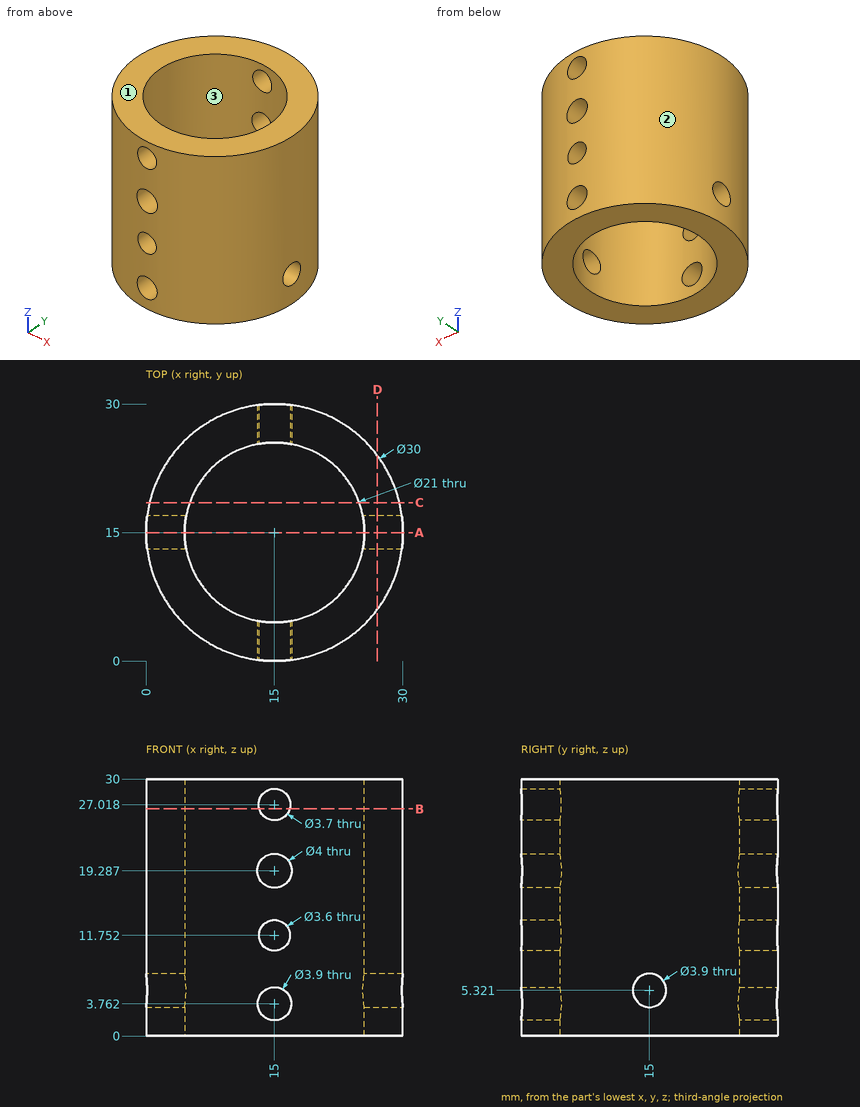
Study the drawing (mm; zero at the part's minimum x, y, z) and answer. Give positions to 0.01 mm unless a question says otherwise; leave off trailing zeros. Loops run counter-clockwise (first coordinate to the right, second up) from the corner with the lowest first, then second, coordinate; pieces in that order, holes last. Notation, with made-up numbers: (38.25, 78.25) -> (89.25, 78.25) arc R33 ccw to (89.25, 110.25) -> close; hole circle Ø7 at (-23.5, 35). An arc over 180 degrees is marked (long way). Write item = value, one per line. Start each with the question number.
(1) The mould has two halves that part along Y. Classify the marked faces 1, 2 and 3: +Y half, -Y half, draft (parallel to the pull), parting line (faces both ways), or undercut.
(2) Given pin 1 Ø12 at (y, z) = (7, 21) entering from -X; pin 2 Ø5 at (y, z) = (7, 17.5) entering from +X (1 decimal); pin 3 Ø1 at (x, z) = (9.5, 17.5) entering from -Y, each flat-ended and moving along its own axis, determine where each tip first touches the part or whether it passes through.
(3) Find the intervals of material crossed by probe 1 along X at (y, z) = (7, 21.5); probe 2 along X at (y, z) = (18.5, 22.5) (1 decimal); probe 3 along Y at (x, z) = (2.5, 4) (1 decimal), in increasing order. Write a range as from..to.
(4) Find section C-C on y = 18.5. Give the vertices of the cut face in (x, z).
(5) Find section B-B on z = 26.5. Give the vertices of the cut face in (x, y) (1 decimal).
(6) Find section A-A on y = 15. Give the vertices of the cut face in (x, z).
(7) Find section D-D on x = 27. Give the vertices of the cut face in (y, z), and give its area (3 significant figures).
From the geometry:
q1.face_1 = draft
q1.face_2 = parting line
q1.face_3 = undercut
q2.pin_1 = 0.13
q2.pin_2 = 29
q2.pin_3 = 0.86
q3.probe_1 = 2.31..8.2, 21.8..27.69
q3.probe_2 = 0.4..5.1, 24.9..29.6
q3.probe_3 = 6.7..13.6, 16.4..23.3
q4.outline = (0.41, 0) -> (5.1, 0) -> (5.1, 30) -> (0.41, 30) -> close; (24.9, 0) -> (29.59, 0) -> (29.59, 30) -> (24.9, 30) -> close
q5.outline = (13.2, 0.1) -> (13.2, 4.7) arc R10.5 cw to (13.2, 25.3) -> (13.2, 29.9) arc R15 ccw to start; (16.8, 0.1) arc R15 ccw to (16.8, 29.9) -> (16.8, 25.3) arc R10.5 cw to (16.8, 4.7) -> close
q6.outline = (0, 0) -> (4.5, 0) -> (4.5, 3.37) -> (0, 3.37) -> close; (0, 7.27) -> (4.5, 7.27) -> (4.5, 30) -> (0, 30) -> close; (25.5, 0) -> (30, 0) -> (30, 3.37) -> (25.5, 3.37) -> close; (25.5, 7.27) -> (30, 7.27) -> (30, 30) -> (25.5, 30) -> close
q7.outline = (6, 0) -> (24, 0) -> (24, 30) -> (6, 30) -> close; hole circle Ø3.9 at (15, 5.32)
q7.area = 528 mm^2
